Job drawing, mm, ordinate dimensions from the low corner. One solid piece. A direction names the side the tool comes from. Round coordinates to 2 decimals unless told otherwise and drop trailing zeros. Loops run counter-clockwise (first coordinate to the right, second up) from the corner with the lowest first, then second, coordinate; pieces in that order, holes last.
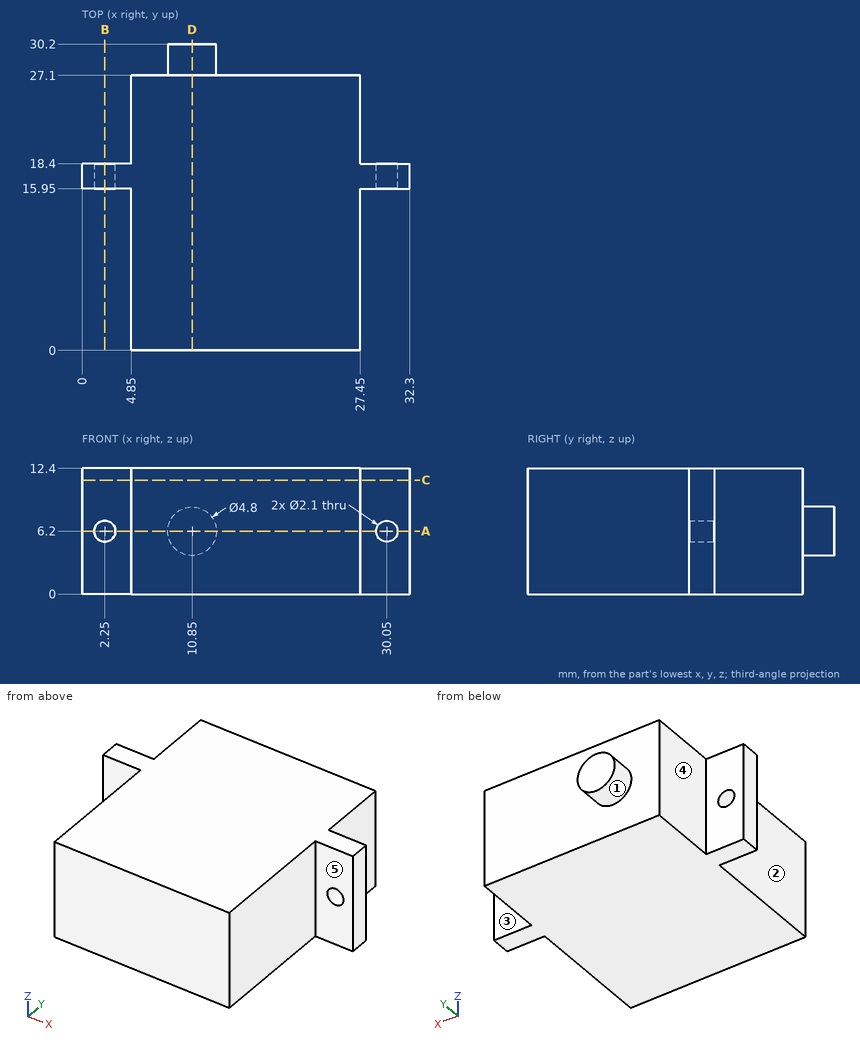
1) Tool access for the marked faces 1, 2, 3, 4 and 5: list every direction of +Z, -Z, +X, -X, +Y, -Y with a clear straight run to the whole face (end or side of a thin tool).
Values:
face 1: +Y
face 2: +Z, -Z, -X, -Y
face 3: +Z, -Z, +X, +Y
face 4: +Z, -Z, -X, +Y
face 5: +Z, -Z, +X, -Y
2) Slice it at A-A, the plane z = 6.2. Give the cut face in (x, y).
Values:
outline: (0, 15.95) - (1.2, 15.95) - (1.2, 18.4) - (0, 18.4) - close; (3.3, 15.95) - (4.85, 15.95) - (4.85, 0) - (27.45, 0) - (27.45, 15.95) - (29, 15.95) - (29, 18.4) - (27.45, 18.4) - (27.45, 27.1) - (13.25, 27.1) - (13.25, 30.2) - (8.45, 30.2) - (8.45, 27.1) - (4.85, 27.1) - (4.85, 18.4) - (3.3, 18.4) - close; (31.1, 15.95) - (32.3, 15.95) - (32.3, 18.4) - (31.1, 18.4) - close
3) Drop flat-ended pins along their axis: pin 1 Ø1.3 at (x, z) = (2.25, 6.2) entering from -Y; pin 2 Ø1.5 at (x, z) = (3, 7.5) entering from +Y; pin 3 Ø2.5 at (y, z) = (24, 8) entering from -X; pin 4 Ø1.5 at (x, z) = (3, 9) entering from -Y. Give the stop position or say it passes through.
Values:
pin 1: passes through
pin 2: stops at y = 18.4
pin 3: stops at x = 4.85
pin 4: stops at y = 15.95
4) Wall check: line 1 along X through (y, z) = (17.35, 6.2); line 2 along Z through (x, y) = (30, 16); line 3 along Y through (x, z) = (19, 11.75). Give the ranges that are in metal, low to high.
Values:
line 1: x = 0 to 1.2, 3.3 to 29, 31.1 to 32.3
line 2: z = 0 to 5.15, 7.25 to 12.4
line 3: y = 0 to 27.1
5) Slice it at D-D, the plane x = 10.85. Give the cut face in (y, z), then the cut area to 3 significant figures.
Values:
outline: (0, 0) - (27.1, 0) - (27.1, 3.8) - (30.2, 3.8) - (30.2, 8.6) - (27.1, 8.6) - (27.1, 12.4) - (0, 12.4) - close
area: 351 mm2
6) Slice it at C-C, the plane z = 11.25. Give the cut face in (x, y), then the cut area to 3 significant figures.
Values:
outline: (0, 15.95) - (4.85, 15.95) - (4.85, 0) - (27.45, 0) - (27.45, 15.95) - (32.3, 15.95) - (32.3, 18.4) - (27.45, 18.4) - (27.45, 27.1) - (4.85, 27.1) - (4.85, 18.4) - (0, 18.4) - close
area: 636 mm2
7) Slice it at B-B, the plane x = 2.25. Give the cut face in (y, z).
Values:
outline: (15.95, 0) - (18.4, 0) - (18.4, 5.15) - (15.95, 5.15) - close; (15.95, 7.25) - (18.4, 7.25) - (18.4, 12.4) - (15.95, 12.4) - close
